from build123d import *

# Parameters (mm, degrees)
SKETCH1_W               = 209.55
SKETCH1_H               = 101.6
BOSS_EXTRUDE1_DEPTH     = 1.5
CUT_EXTRUDE1_DEPTH      = 117.479357077
CUT_EXTRUDE1_DEPTH_BACK = 117.479357077
SKETCH2_R               = 311.15
CUT_EXTRUDE2_DEPTH      = 117.479357077
CUT_EXTRUDE2_DEPTH_BACK = 117.479357077
CUT_EXTRUDE3_DEPTH      = 117.479357077
CUT_EXTRUDE3_DEPTH_BACK = 117.479357077
SKETCH5_W               = 3
SKETCH5_H               = 6.096


with BuildPart() as part:
    # Sketch1 → Boss-Extrude1 (new, symmetric)
    with BuildSketch(Plane(origin=(0, 0, 0), x_dir=(1, 0, 0), z_dir=(0, 1, 0))):
        Rectangle(SKETCH1_W, SKETCH1_H)
    extrude(amount=BOSS_EXTRUDE1_DEPTH, both=True)

    # Sketch2 → Cut-Extrude1 (cut, two sides: drawn at the far end of the back side and taken through both)
    with BuildSketch(Plane(origin=(0, 1.5, 0), x_dir=(1, 0, 0), z_dir=(0, 1, 0)).offset(-CUT_EXTRUDE1_DEPTH_BACK)):
        with Locations((0, -336.55)):
            Circle(SKETCH2_R)
    extrude(amount=CUT_EXTRUDE1_DEPTH + CUT_EXTRUDE1_DEPTH_BACK, mode=Mode.SUBTRACT)

    # Sketch4 → Cut-Extrude2 (cut, two sides: drawn at the far end of the back side and taken through both)
    with BuildSketch(Plane(origin=(0, 1.5, 0), x_dir=(1, 0, 0), z_dir=(0, 1, 0)).offset(-CUT_EXTRUDE2_DEPTH_BACK)):
        Polygon((47.625, -29.066371371), (47.625, -3.666371371), (104.775, -3.666371371), (104.775, -43.571294502), align=None)
    extrude(amount=CUT_EXTRUDE2_DEPTH + CUT_EXTRUDE2_DEPTH_BACK, mode=Mode.SUBTRACT)

    # Sketch5 → Cut-Extrude3 (cut, two sides: drawn at the far end of the back side and taken through both)
    with BuildSketch(Plane(origin=(0, 1.5, 0), x_dir=(1, 0, 0), z_dir=(0, 1, 0)).offset(-CUT_EXTRUDE3_DEPTH_BACK)):
        with Locations((87.733, 44.577)):
            Rectangle(SKETCH5_W, SKETCH5_H)
        with Locations((87.733, 31.877)):
            Rectangle(SKETCH5_W, SKETCH5_H)
        with Locations((87.733, 19.177)):
            Rectangle(SKETCH5_W, SKETCH5_H)
        with Locations((87.733, 6.477)):
            Rectangle(SKETCH5_W, SKETCH5_H)
        with Locations((62.333, 31.877)):
            Rectangle(SKETCH5_W, SKETCH5_H)
        with Locations((62.333, 19.177)):
            Rectangle(SKETCH5_W, SKETCH5_H)
        with Locations((62.333, 6.477)):
            Rectangle(SKETCH5_W, SKETCH5_H)
        with Locations((62.333, 44.577)):
            Rectangle(SKETCH5_W, SKETCH5_H)
    extrude(amount=CUT_EXTRUDE3_DEPTH + CUT_EXTRUDE3_DEPTH_BACK, mode=Mode.SUBTRACT)


solid = part.part
Model file for the job. Use its own axes, mm. Coordinates: 2 decimals unless noted, no trailing zeros. Order: outer loops, then holes, each group sorted by start corner. A loop starts at its lowest first (then second) coordinate and runs counter-clockwise, first axis right, second up. Notation, with made-up numbers: (61.25, -15) -> (71.25, -15) arc R17 cw to (71.25, 15) -> close; hole circle Ø4 at (58, 65). An arc over 180 degrees is marked (long way). Return JSON: item names as keys, results as strings. Group by question number.
Item 1: Pull direction X, two halves, no side cores. Call faces 1 (the cylindrical face through (-28.4, 0, 26.7)), 2 (the flat face through (-1, -1.5, -15)): pulls with the +X half, pulls with the -X half, needs draft (parallel to the pull), parting line crosses it, or undercut.
Item 2: Saw through at B-B on y = -0.3. State how many separate pieces and enclosed holes the cut face has, then the cut area to 3 significant figures.
Item 3: Flat gauge pins, fed straight in: P1, Ø1.5, axis at x = 88, y = 0.5, coming from the +Z side; P2, Ø10, axis at x = -33, z = 27.5, coming from the +Y side; P3, Ø0.9, axis at y = -0.5, z = 15.5, coming from the +X side (3 decimals). Where does each tip first touch, or does it go through?
Item 4: Saw through at C-C on z = 6. Write the cut outline in (x, y) (3 decimals).
Item 5: Saw through at A-A on x = 78. Write the cut outline in (y, z).
Item 6: Wall check: line 1 along X through (y, z) = (-0.5, -7) (3 decimals); line 2 along Z through (x, y) = (61, -1.2) (3 decimals); line 3 along Z through (x, y) = (68, 0.75). Give the ranges that are in metal, low to high. Write a range as [from, to].
Values found:
{
 "1": {"face 1": "undercut", "face 2": "needs draft"},
 "2": {"separate pieces": "1", "enclosed holes": "8", "area": "15,300 mm2"},
 "3": {"P1": "stops at z = 3.67", "P2": "stops at y = 1.5", "P3": "stops at x = 47.625"},
 "4": {"outline": "(-104.775, -1.5) -> (47.625, -1.5) -> (47.625, 1.5) -> (-104.775, 1.5) -> close"},
 "5": {"outline": "(-1.5, -50.8) -> (1.5, -50.8) -> (1.5, 3.67) -> (-1.5, 3.67) -> close"},
 "6": {"line 1": "x = [-104.775, 60.833], [63.833, 86.233], [89.233, 104.775]", "line 2": "z = [-50.8, -47.625], [-41.529, -34.925], [-28.829, -22.225], [-16.129, -9.525], [-3.429, 3.666]", "line 3": "z = [-50.8, 3.67]"}
}
